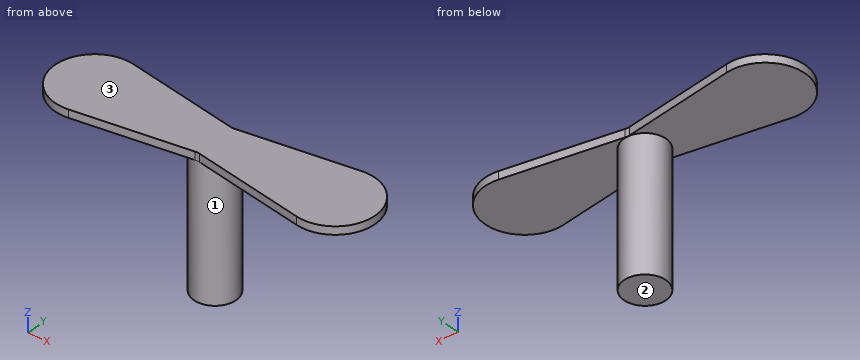
from build123d import *

# Parameters (mm, degrees)
SKETCH1_R           = 7.9375
BOSS_EXTRUDE1_DEPTH = 50
BOSS_EXTRUDE2_DEPTH = 3
FILLET1_R           = 5


with BuildPart() as part:
    # Sketch1 → Boss-Extrude1 (new body)
    with BuildSketch(Plane.XY):
        Circle(SKETCH1_R)
    extrude(amount=BOSS_EXTRUDE1_DEPTH)

    # Sketch2 → Boss-Extrude2 (add)
    with BuildSketch(Plane.XY.offset(50)):
        with BuildLine():
            Line((0, -7.9375), (0, 7.9375))
            Line((0, 7.9375), (42.612091922, 14.808710106))
            ThreePointArc((42.612091922, 14.808710106), (60, 0), (42.612091922, -14.808710106))
            Line((42.612091922, -14.808710106), (0, -7.9375))
        make_face()
    boss_extrude2 = extrude(amount=BOSS_EXTRUDE2_DEPTH)

    # Mirror1: Boss-Extrude2 across plane
    add(boss_extrude2.mirror(Plane(origin=(0, -7.9375, 53), x_dir=(0, 0, 1), z_dir=(1, 0, 0))))

    # Fillet1
    fillet1_edges = [part.edges().sort_by_distance(p)[0] for p in [
        (0, 7.9375, 51.5),
        (0, -7.9375, 51.5),
    ]]
    fillet(fillet1_edges, radius=FILLET1_R)


solid = part.part
The model under review builds one solid part; all positions refer to its coordinate system, in mm. Face numbers are marked on the shaded views. Give positions to 0.01 mm unless a question says otherwise; leave off trailing zeros. Loops run counter-clockwise (first coordinate to the right, second up) from the corner with the lowest first, then second, coordinate; pieces in that order, holes last. Notation, with made-up numbers: (-7.5, 43) -> (12.5, 43) arc R13 cw to (12.5, 57) -> close; hole circle Ø1 at (-3.75, -24). An arc over 180 degrees is marked (long way). Write each question's results on one line, items separated by ' | '.
1) Take a section at B-B, the plane y = -11. Give the boundary of the cut face in (x, z), plus the area to 3 significant figures.
Conclusion:
outline: (-55.2, 50) -> (-18.99, 50) -> (-18.99, 53) -> (-55.2, 53) -> close; (18.99, 50) -> (55.2, 50) -> (55.2, 53) -> (18.99, 53) -> close | area: 217 mm^2
2) Take a section at C-C, the plane z = 11.5. Give the boundary of the cut face in (x, y) (1 decimal).
Conclusion:
outline: circle Ø15.9 at (0, 0)
3) Take a section at A-A, the plane y = 0. Give the boundary of the cut face in (x, z), plus the area to 3 significant figures.
Conclusion:
outline: (-60, 50) -> (-7.94, 50) -> (-7.94, 0) -> (7.94, 0) -> (7.94, 50) -> (60, 50) -> (60, 53) -> (-60, 53) -> close | area: 1,150 mm^2
4) For line 1 along Z through (x, y) = (-49, -8); line 2 along X through (y, z) = (6, 39.5); line 3 along X through (y, z) = (2.5, 12.5), list the stretches that pass through material, from the lowest coordinate up. Write a range as from..to.
Conclusion:
line 1: z = 50..53 | line 2: x = -5.2..5.2 | line 3: x = -7.53..7.53
5) Insertion check: pin 1 Ø10 at (y, z) = (4.5, 35) entering from -X; pin 2 Ø2 at (y, z) = (10, 19.5) entering from +X; pin 3 Ø12 at (x, y) = (45.5, -3) entering from -Z; pin 4 Ø1.5 at (x, z) = (0.5, 14.5) entering from -Y. Each pin has a flat end and moves straight along its axis. Give the tip position at first contact, or say it passes through.
Conclusion:
pin 1: stops at x = -7.94 | pin 2: passes through | pin 3: stops at z = 50 | pin 4: stops at y = -7.94
6) Take a section at D-D, the plane x = -45. Give the boundary of the cut face in (y, z).
Conclusion:
outline: (-15, 50) -> (15, 50) -> (15, 53) -> (-15, 53) -> close
7) Draft analysis for pull direction Z (two halves, no side actions). For the marked faces 1, 2 and 3, state which applies: pulls with the +Z half, pulls with the -Z half, needs draft (parallel to the pull), parting line crosses it, or undercut.
Conclusion:
face 1: needs draft | face 2: pulls with the -Z half | face 3: pulls with the +Z half
